from build123d import *

# Parameters (mm, degrees)
SKETCH_1_W          = 53
SKETCH_1_H          = 17.5
EXTRUDE_1_DEPTH     = 2
SKETCH_3_W          = 51
SKETCH_3_H          = 15.5
CUT_EXTRUDE_2_DEPTH = 0.5
SKETCH_2_W          = 48
SKETCH_2_H          = 12.5
CUT_EXTRUDE_3_DEPTH = 2
FILLET_1_R          = 1
SKETCH_5_W          = 0.1
SKETCH_5_H          = 15.5
CUT_EXTRUDE_5_DEPTH = 28.978786607


with BuildPart() as part:
    # Эскиз1 → Бобышка-Вытянуть1 (new, symmetric)
    with BuildSketch(Plane.XY):
        Rectangle(SKETCH_1_W, SKETCH_1_H)
    extrude(amount=EXTRUDE_1_DEPTH, both=True)

    # Эскиз3 → Вырез-Вытянуть2 (cut, symmetric)
    with BuildSketch(Plane.XY):
        Rectangle(SKETCH_3_W, SKETCH_3_H)
    extrude(amount=CUT_EXTRUDE_2_DEPTH, both=True, mode=Mode.SUBTRACT)

    # Эскиз2 → Вырез-Вытянуть3 (cut)
    with BuildSketch(Plane.XY.offset(2)):
        Rectangle(SKETCH_2_W, SKETCH_2_H)
    extrude(amount=-CUT_EXTRUDE_3_DEPTH, mode=Mode.SUBTRACT)

    # Скругление1
    fillet_1_edges = [part.edges().sort_by_distance(p)[0] for p in [
        (26.5, 0, 2),
        (0, 8.75, 2),
        (-24, 0, 2),
        (0, -6.25, 2),
        (24, 0, 2),
        (0, 6.25, 2),
        (-26.5, 0, 2),
        (0, -8.75, 2),
    ]]
    fillet(fillet_1_edges, radius=FILLET_1_R)

    # Эскиз5 → Вырез-Вытянуть5 (cut, through all)
    with BuildSketch(Plane(origin=(0, 0, 0), x_dir=(0, 0, -1), z_dir=(1, 0, 0))):
        with Locations((-0.05, 0)):
            Rectangle(SKETCH_5_W, SKETCH_5_H)
    extrude(amount=-CUT_EXTRUDE_5_DEPTH, mode=Mode.SUBTRACT)


solid = part.part
The listing builds one solid part. Answer for the finished solid, in the listing's coordinates (mm). A direction names the side the tool comes from. Coordinates: 2 decimals unless noted, no trailing zeros. Loops run counter-clockwise (first coordinate to the right, second up) from the corner with the lowest first, then second, coordinate; pieces in that order, holes last. Notation, with made-up numbers: M 16,53 L 38,53 A29 ccw 38,82 Z; hole C 29.5,34 d11. An arc over 180 degrees is marked long. Answer in a Markdown table with one row per item.
1) Given pin 1 (1.5 mm diameter, centred on x = 2.5, y = 7, fed in from +Z); pin 2 (8 mm diameter, centred on x = 1, y = -2.5, fed in from +Z), each flat-ended and moving along its own axis, determine where each tip first touches the part or whether it passes through.
Answers below:
| item | result |
|---|---|
| pin 1 | z = 2 |
| pin 2 | z = 1.66 |
2) Find the intervals of material crossed by probe 1 along Z at (x, y) = (-19, 7.5); probe 2 along Y at (x, z) = (9, -0.3); probe 3 along X at (y, z) = (-6.5, 0.4), in increasing order.
Answers below:
| item | result |
|---|---|
| probe 1 | -2 to -0.5, 0.5 to 2 |
| probe 2 | -8.75 to -7.75, 7.75 to 8.75 |
| probe 3 | -26.5 to -25.5, 25.5 to 26.5 |
3) Find section A-A (y = -4.75). Determine the outline of the cut face in (x, z).
Answers below:
| item | result |
|---|---|
| outline | M -26.5,-2 L 26.5,-2 L 26.5,1 A1 ccw 25.5,2 L 25,2 A1 ccw 24,1 L 24,0.5 L 25.5,0.5 L 25.5,-0.5 L -25.5,-0.5 L -25.5,0 L -26.5,0 Z; M -26.5,0.1 L -25.5,0.1 L -25.5,0.5 L -24,0.5 L -24,1 A1 ccw -25,2 L -25.5,2 A1 ccw -26.5,1 Z |
4) Which of the six approach directions +Z, -Z, +X, -X, +Y, -Y give full straight-line access (tool end or side, diameter ignored) to faces 1 (the cylindrical face through (24.301, 0.101, 1.715)), 2 (the cylindrical face through (0.371, -8.465, 1.699)), 3 (the flat face through (-0.1, 6.4, 0.5))?
Answers below:
| item | result |
|---|---|
| face 1 | +Z |
| face 2 | +Z, +X, -X, -Y |
| face 3 | none |
5) Find section B-B (x = 2). Determine the outline of the cut face in (y, z).
Answers below:
| item | result |
|---|---|
| outline | M -8.75,-2 L 8.75,-2 L 8.75,1 A1 ccw 7.75,2 L 7.25,2 A1 ccw 6.25,1 L 6.25,0.5 L 7.75,0.5 L 7.75,-0.5 L -7.75,-0.5 L -7.75,0.5 L -6.25,0.5 L -6.25,1 A1 ccw -7.25,2 L -7.75,2 A1 ccw -8.75,1 Z |
6) Determine the mould class of faces 4 (the flat face through (26.5, 0, 0)), 5 (the cylindrical face through (-24.301, 0.101, 1.715)), 6 (the flat face through (-26.5, -0.1, -0.5)) for opening direction X: released by +X, released by -X, zero draft, split by the parting line, or undercut.
Answers below:
| item | result |
|---|---|
| face 4 | released by +X |
| face 5 | undercut |
| face 6 | released by -X |
